Geometry: see drawing. Coordinates: mm, zero at the bounding-box minimum. A direction names the side the tool comes from. Give positions to 0.01 mm unless a question says otherwise; leave off trailing zeros. Order: outer loops, then holes, each group sorted by start corner. A loop starts at its lowest first (then second) coordinate and runs counter-clockwise, first axis right, second up. Notation, with made-up numbers: M 58.25,86.5 L 84.25,86.5 A12 ccw 84.25,105.5 Z; hole C 72.5,83.25 d2. An arc over 180 degrees is marked long. Return JSON: item names as keys, results as strings.
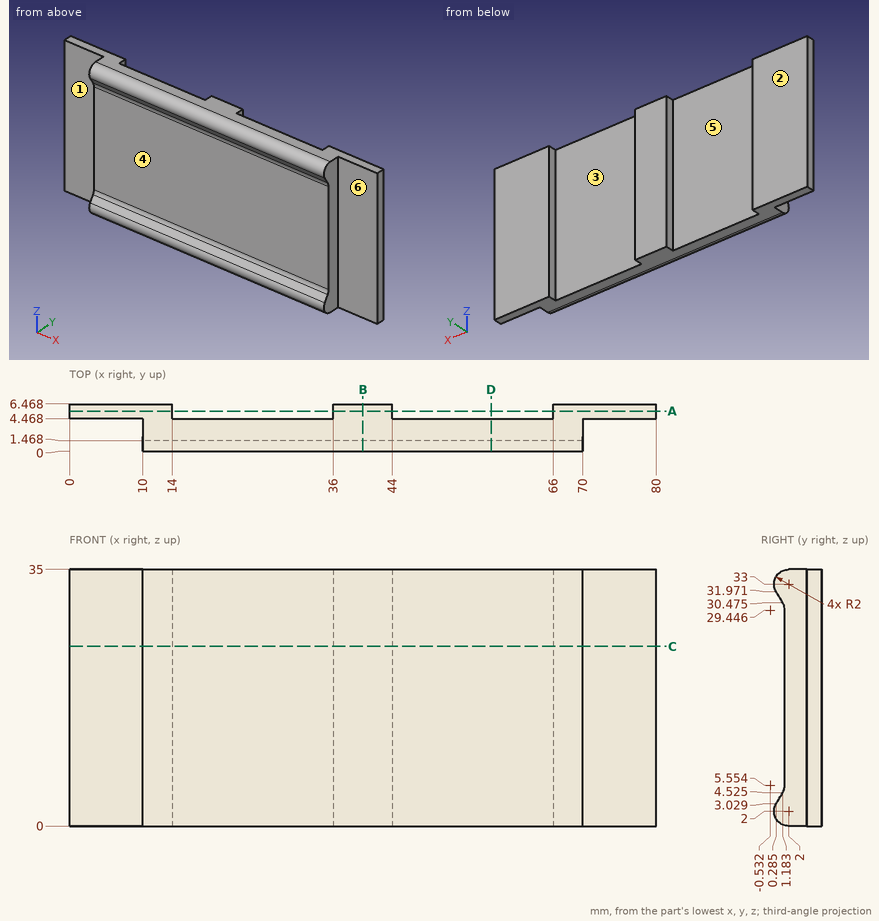
1. Ray query, probe 1 along X at (y, z) = (5, 26); probe 2 along Y at (x, z) = (58.5, 21.5); probe 3 along X at (y, z) = (2.25, 4). Return the intervals inside material, ascending.
Evaluation:
{"probe 1": "x = 0 to 14, 36 to 44, 66 to 80", "probe 2": "y = 1.47 to 4.47", "probe 3": "x = 10 to 70"}
2. Section query C-C (z = 24.5). Return loops of the section in (x, y).
Evaluation:
{"outline": "M 0,4.47 L 10,4.47 L 10,1.47 L 70,1.47 L 70,4.47 L 80,4.47 L 80,6.47 L 66,6.47 L 66,4.47 L 44,4.47 L 44,6.47 L 36,6.47 L 36,4.47 L 14,4.47 L 14,6.47 L 0,6.47 Z"}
3. Section query A-A (y = 5.5). Return loops of the section in (x, z), then the cut area to 3 significant figures.
Evaluation:
{"outline": "M 0,0 L 14,0 L 14,35 L 0,35 Z; M 36,0 L 44,0 L 44,35 L 36,35 Z; M 66,0 L 80,0 L 80,35 L 66,35 Z", "area": "1,260 mm^2"}
4. Section query D-D (x = 57.5). Return loops of the section in (y, z) (1 decimal), then the cut area to 3 significant figures.
Evaluation:
{"outline": "M 0.3,3 A2 ccw 2,0 L 4.5,0 L 4.5,35 L 2,35 A2 ccw 0.3,32 L 1.2,30.5 A2 cw 1.5,29.4 L 1.5,5.6 A2 cw 1.2,4.5 Z", "area": "114 mm^2"}
5. Set-up query: the marked faces 1, 2, 3 and 4. Return all of +Z, -Z, +X, -X, +Y, -Y with unobstructed straight access to the full face (end or side cutting, diameter ignored); none if empty.
Evaluation:
{"face 1": "+Z, -Z, -X, -Y", "face 2": "+Z, -Z, +X, -X, +Y", "face 3": "+Z, -Z, +Y", "face 4": "+X, -X, -Y"}
6. Draft query along X for the marked faces 5 and 6. Return one class per face: pulls with the +X half, pulls with the -X half, needs draft (parallel to the pull), parting line crosses it, or undercut.
Evaluation:
{"face 5": "undercut", "face 6": "needs draft"}
7. Section query B-B (x = 40). Return loops of the section in (y, z) (1 decimal), then the cut area to 3 significant figures.
Evaluation:
{"outline": "M 0.3,3 A2 ccw 2,0 L 6.5,0 L 6.5,35 L 2,35 A2 ccw 0.3,32 L 1.2,30.5 A2 cw 1.5,29.4 L 1.5,5.6 A2 cw 1.2,4.5 Z", "area": "184 mm^2"}
8. First-contact query: pin 1 (3.5 mm diameter, centred on y = 1.5, z = 16, fed in from -X); pin 2 (6.5 mm diameter, centred on x = 56, z = 23.5, fed in from +Y); pin 3 (2 mm diameter, centred on y = 2, z = 21.5, fed in from +X). Flat tips, straight axial feed; report the tip coordinate or a pass-through.
Evaluation:
{"pin 1": "stops at x = 10", "pin 2": "stops at y = 4.47", "pin 3": "stops at x = 70"}
